Source: CAD feature listing. Evaluate the final solid. Frame: model axes, mm. Give positions to 0.01 mm unless a question says otherwise; leave off trailing zeros. Loops run counter-clockwise (first coordinate to the right, second up) from the corner with the lowest first, then second, coordinate; pieces in that order, holes last. Notation, with made-up numbers: (-23, 49.25) -> (-19, 49.25) arc R17 ccw to (-19, 65.25) -> close; hole circle Ø11 at (-8.5, 87). An arc over 180 degrees is marked (long way). Return JSON: item names as keys, results as strings. Group by question number.
Autodesk Inventor part; units mm, degrees
ref_plane "YZ Plane" through (0, 0, 0) normal (1, 0, 0) x (0, 1, 0)
ref_plane "XZ Plane" through (0, 0, 0) normal (0, 1, 0) x (-1, 0, 0)
ref_plane "XY Plane" through (0, 0, 0) normal (0, 0, 1) x (1, 0, 0)
sketch "Sketch1" plane through (0, 0, 0) normal (0, 1, 0) x (-1, 0, 0)
  line L0 (0, 0) -> (10, 0)
  line L1 (10, 0) -> (10, -10)
  line L2 (10, -10) -> (0, -10)
  line L3 (0, -10) -> (0, 0)
  dimension "d0" = 10
  dimension "d1" = 10
extrude "Extrusion1" add sketch "Sketch1" along normal blind 100
sketch "Sketch2" plane through (0, 0, 0) normal (1, 0, 0) x (0, 0, -1)
  circle A0 centre (5, 95) radius 3
  line L0 (10, 0) -> (10, 100)
  line L1 (0, 100) -> (10, 100)
  line L2 (0, 0) -> (10, 0)
  line L3 (10, 0) -> (10, 100)
  line L4 (0, 100) -> (10, 100)
  line L5 (0, 0) -> (0, 100)
  circle A1 centre (5, 85) radius 3
  circle A2 centre (5, 75) radius 3
  circle A3 centre (5, 65) radius 3
  circle A4 centre (5, 55) radius 3
  circle A5 centre (5, 45) radius 3
  circle A6 centre (5, 35) radius 3
  circle A7 centre (5, 25) radius 3
  circle A8 centre (5, 15) radius 3
  circle A9 centre (5, 5) radius 3
  line L6 (0, 0) -> (0, 100)
  line L7 (10, 0) -> (10, 100)
  arc A10 (0, 5) -> (10, 5) centre (5, 5) ccw
  line L8 (10, 0) -> (0, 0)
  point P0 (5, 0)
  point P1 (0, 5)
  point P2 (10, 5)
  dimension "d4" = 6
  dimension "d5" = 5
  dimension "d6" = 5
  dimension "d9" = 10
extrude "Extrusion2" cut sketch "Sketch2" against normal through all contours A0 | L2 A10 L0 | L2 L5 A10 | A1 | A2 | A3 | A4 | A5 | A6 | A7 | A8 | A9
fillet "Fillet1" radius 1 6 edges at (0, 0, -5) (0, 52.5, -10) (0, 52.5, 0) (-10, 0, -5) (-10, 52.5, -10) (-10, 52.5, 0)
properties part number "Stang3D"
1) Cut plane C-C on y = 53. Return loops of the section in (x, z).
2) Mould query, pull axis Y, two halves, no side actions, for faces 1 (the face through (-5, 58, -5)), 2 (the face through (-5, 100, -5)), 3 (the face through (-4.9, 23.2, -2.6)), 4 (the face through (-5, 52, 0)). Classes: released by +Y, released by -Y, zero draft, split by the parting line, or undercut.
3) Material intervals for line 1 (Z direction, x = -8.5, y = 84); line 2 (Y direction, x = -6.75, z = -9); line 3 (Z direction, x = -4.5, y = 77), sorted ascending.
4) Contact query for flat-ended pins moving along their axis: P1, Ø1.5, axis at x = -2.5, z = -8.5, coming from the -Y side; P2, Ø3.5, axis at y = 15, z = -5, coming from the +X side. Output: stop coordinate, or through.
5) Cut plane A-A on y = 25. Return loops of the section in (x, z).
6) Cut plane B-B on x = -2. Count the separate pieces of the cut face and the enclosed holes in it, then the cut area to 3 significant figures.
Calculated:
{
 "1": {"outline": "(-10, -9) arc R1 ccw to (-9, -10) -> (-1, -10) arc R1 ccw to (0, -9) -> (0, -7.24) -> (-10, -7.24) -> close; (-10, -2.76) -> (0, -2.76) -> (0, -1) arc R1 ccw to (-1, 0) -> (-9, 0) arc R1 ccw to (-10, -1) -> close"},
 "2": {"face 1": "undercut", "face 2": "released by +Y", "face 3": "undercut", "face 4": "zero draft"},
 "3": {"line 1": "-10 to -7.83, -2.17 to 0", "line 2": "2 to 100", "line 3": "-10 to -7.24, -2.76 to 0"},
 "4": {"P1": "y = 0.82", "P2": "through"},
 "5": {"outline": "(-10, -9) arc R1 ccw to (-9, -10) -> (-1, -10) arc R1 ccw to (0, -9) -> (0, -8) -> (-10, -8) -> close; (-10, -2) -> (0, -2) -> (0, -1) arc R1 ccw to (-1, 0) -> (-9, 0) arc R1 ccw to (-10, -1) -> close"},
 "6": {"separate pieces": "1", "enclosed holes": "10", "area": "707 mm2"}
}
